Input: part model. Units: mm. Frame: model coordinates. Face numbers are marked on the shaded views. A direction names the side the tool comes from. Round coordinates to 2 decimals unless told otherwise and drop trailing zeros. Write each loop counter-clockwise with the first axis right and the second up, starting at its lowest first coordinate (ties: lowest second). Pieces come first, ordered by that corner, then holes. Notation, with made-up numbers: (59.5, 70.25) -> (69.5, 70.25) arc R7 ccw to (69.5, 77.25) -> close; hole circle Ø1 at (80.25, 30). An arc over 180 degrees is marked (long way). Write item = value, one per line.
Autodesk Inventor part; units mm, degrees
ref_plane "YZ Plane" through (0, 0, 0) normal (1, 0, 0) x (0, 1, 0)
ref_plane "XZ Plane" through (0, 0, 0) normal (0, 1, 0) x (-1, 0, 0)
ref_plane "XY Plane" through (0, 0, 0) normal (0, 0, 1) x (1, 0, 0)
sketch "Skizze1" plane through (0, 0, 0) normal (0, 0, 1) x (1, 0, 0)
  circle A0 centre (0, 0) radius 5
  dimension "d0" = 10
extrude "Extrusion1" add sketch "Skizze1" along normal blind 1
sketch "Skizze2" plane through (0, 0, 1) normal (0, 0, 1) x (1, 0, 0)
  circle A0 centre (0, 0) radius 5
  circle A1 centre (0, 0) radius 7.5
  circle A2 centre (0, 0) radius 5
  line L0 (0, -5) -> (-1.3746, -7.373)
  line L1 (-1.3746, -7.373) -> (-1.8625, -4.6402)
  arc A3 (-1.8625, -4.6402) -> (0, -5) centre (0, 0) ccw
  line L2 (2.1694, -4.5048) -> (1.9606, -7.2392)
  line L3 (1.9606, -7.2392) -> (0.3352, -4.9888)
  arc A4 (0.3352, -4.9888) -> (2.1694, -4.5048) centre (0, 0) ccw
  line L4 (3.9092, -3.1174) -> (4.9074, -5.6716)
  line L5 (4.9074, -5.6716) -> (2.4666, -4.3493)
  arc A5 (2.4666, -4.3493) -> (3.9092, -3.1174) centre (0, 0) ccw
  line L6 (4.8746, -1.1126) -> (6.8822, -2.9807)
  line L7 (6.8822, -2.9807) -> (4.1094, -2.8484)
  arc A6 (4.1094, -2.8484) -> (4.8746, -1.1126) centre (0, 0) ccw
  line L8 (4.8746, 1.1126) -> (7.494, 0.3005)
  line L9 (7.494, 0.3005) -> (4.9383, -0.7833)
  arc A7 (4.9383, -0.7833) -> (4.8746, 1.1126) centre (0, 0) ccw
  line L10 (3.9092, 3.1174) -> (6.6214, 3.5223)
  line L11 (6.6214, 3.5223) -> (4.7891, 1.4369)
  arc A8 (4.7891, 1.4369) -> (3.9092, 3.1174) centre (0, 0) ccw
  line L12 (2.1694, 4.5048) -> (4.4375, 6.0464)
  line L13 (4.4375, 6.0464) -> (3.6914, 3.3725)
  arc A9 (3.6914, 3.3725) -> (2.1694, 4.5048) centre (0, 0) ccw
  line L14 (0, 5) -> (1.3746, 7.373)
  line L15 (1.3746, 7.373) -> (1.8625, 4.6402)
  arc A10 (1.8625, 4.6402) -> (0, 5) centre (0, 0) ccw
  line L16 (-2.1694, 4.5048) -> (-1.9606, 7.2392)
  line L17 (-1.9606, 7.2392) -> (-0.3352, 4.9888)
  arc A11 (-0.3352, 4.9888) -> (-2.1694, 4.5048) centre (0, 0) ccw
  line L18 (-3.9092, 3.1174) -> (-4.9074, 5.6716)
  line L19 (-4.9074, 5.6716) -> (-2.4666, 4.3493)
  arc A12 (-2.4666, 4.3493) -> (-3.9092, 3.1174) centre (0, 0) ccw
  line L20 (-4.8746, 1.1126) -> (-6.8822, 2.9807)
  line L21 (-6.8822, 2.9807) -> (-4.1094, 2.8484)
  arc A13 (-4.1094, 2.8484) -> (-4.8746, 1.1126) centre (0, 0) ccw
  line L22 (-4.8746, -1.1126) -> (-7.494, -0.3005)
  line L23 (-7.494, -0.3005) -> (-4.9383, 0.7833)
  arc A14 (-4.9383, 0.7833) -> (-4.8746, -1.1126) centre (0, 0) ccw
  line L24 (-3.9092, -3.1174) -> (-6.6214, -3.5223)
  line L25 (-6.6214, -3.5223) -> (-4.7891, -1.4369)
  arc A15 (-4.7891, -1.4369) -> (-3.9092, -3.1174) centre (0, 0) ccw
  line L26 (-2.1694, -4.5048) -> (-4.4375, -6.0464)
  line L27 (-4.4375, -6.0464) -> (-3.6914, -3.3725)
  arc A16 (-3.6914, -3.3725) -> (-2.1694, -4.5048) centre (0, 0) ccw
  dimension "d3" = 15
  dimension "d6" = 360
extrude "Extrusion2" add sketch "Skizze2" along normal blind 10 contours A0 | A0 L8 L9 | A0 L10 L11 | L6 L7 A0 | A0 L12 L13 | L4 L5 A0 | L15 A0 L14 | L3 A0 L2 | L17 A0 L16 | L1 A0 L0 | L19 A0 L18 | L27 A0 L26 | L21 A0 L20 | L25 A0 L24 | L23 A0 L22
equation "\"d0\" = Durchmesser3"
equation "\"d3\" = Durchmesser1"
equation "\"Durchmesser1\" = 15"
equation "\"Größe1\" = 7"
equation "\"Durchmesser2\" = 3"
equation "\"Durchmesser3\" = 10"
equation "\"Größe3\" = 3"
equation "\"Größe4\" = 15"
properties part number "WelleRuder"
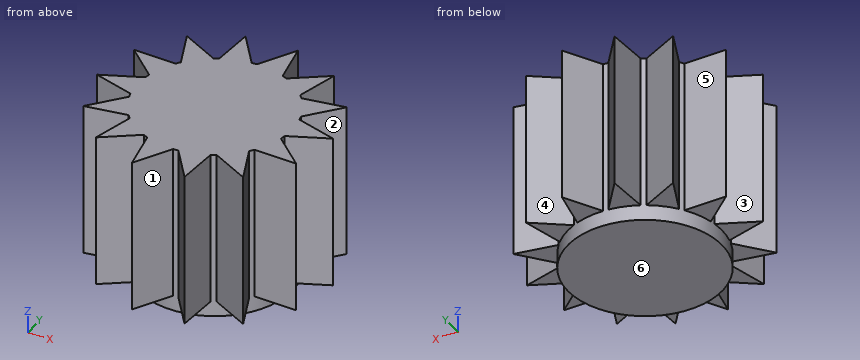
1) Cut plane B-B (y = 0). Return the cut outline in (x, z), and give its area (3 significant figures).
Solutions:
outline = (-6.79, 1) -> (-5, 1) -> (-5, 0) -> (5, 0) -> (5, 1) -> (6.79, 1) -> (6.79, 11) -> (-6.79, 11) -> close
area = 146 mm^2
2) Line query: L1, parallel to Y at x = 5.5, z = 10.5; L2, parallel to Y at x = -5.5, z = 8.25; L3, parallel to X at y = -6.5, z = 2.75. Output: solid intervals per line, ascending. Write a range as from..to.
Solutions:
L1 = -2.91..-1.69, -0.55..0.92, 2.25..3.35
L2 = -3.35..-2.25, -0.92..0.55, 1.69..2.91
L3 = -1.53..-0.87, 1.43..2.02
3) First-contact query: P1, Ø1.5, axis at x = -6, y = 0, coming from the -Z side; P2, Ø1, axis at y = 0.5, z = 7, coming from the +X side. Flat tips, straight axial feed; report the tip coordinate or a pass-through.
Solutions:
P1 = 1
P2 = 7.49
4) Access query for the marked faces 1, 2 and 3. Directions: +Z, -Z, +X, -X, +Y, -Y. A direction counts if a zero-diameter tool reaches every point of the face in a straight line with its end or side. Return the directions, or none.
Solutions:
face_1 = +Z, -Z, -Y
face_2 = +Z, -Z, +X
face_3 = +Z, -Z, -X
5) Cut plane A-A (x = 5.5). Return the cut outline in (y, z), and give its area (3 significant figures).
Solutions:
outline = (-2.91, 1) -> (-1.69, 1) -> (-1.69, 11) -> (-2.91, 11) -> close; (-0.55, 1) -> (0.92, 1) -> (0.92, 11) -> (-0.55, 11) -> close; (2.25, 1) -> (3.35, 1) -> (3.35, 11) -> (2.25, 11) -> close
area = 37.9 mm^2
6) Draft query along Y for the marked faces 4, 5 and 6. Return one class per face: +Y half, -Y half, draft (parallel to the pull), parting line (faces both ways), or undercut.
Solutions:
face_4 = +Y half
face_5 = undercut
face_6 = draft
7) Cut plane C-C (x = -3.5). Return the cut outline in (y, z).
Solutions:
outline = (-5.41, 1) -> (-3.57, 1) -> (-3.57, 0) -> (3.57, 0) -> (3.57, 1) -> (4.91, 1) -> (4.91, 11) -> (-5.41, 11) -> close
